Source: CAD feature listing. Evaluate the final solid. Frame: model axes, mm. A direction names the side the tool comes from. Coordinates: 2 decimals unless noted, no trailing zeros. Order: outer loops, then holes, each group sorted by start corner. A loop starts at its lowest first (then second) coordinate and runs counter-clockwise, first axis right, second up.
```python
from build123d import *

# Parameters (mm, degrees)
SKETCH2_W            = 45.5
SKETCH2_H            = 21
BOSS_EXTRUDE2_DEPTH  = 2
SKETCH4_R            = 8
BOSS_EXTRUDE3_DEPTH  = 12.5
SKETCH5_R            = 6
CUT_EXTRUDE1_DEPTH   = 2.5
BOSS_EXTRUDE5_DEPTH  = 4
SKETCH7_W            = 6
SKETCH7_H            = 3
BOSS_EXTRUDE6_DEPTH  = 3
SKETCH8_W            = 1
SKETCH8_H            = 1
BOSS_EXTRUDE7_DEPTH  = 1
SKETCH10_W           = 1
SKETCH10_H           = 0.8
BOSS_EXTRUDE8_DEPTH  = 6
SKETCH11_R           = 1
CUT_EXTRUDE2_DEPTH   = 15.5
BOSS_EXTRUDE10_DEPTH = 0.1


with BuildPart() as part:
    # Sketch2 → Boss-Extrude2 (new body)
    with BuildSketch(Plane(origin=(0, 0, 0), x_dir=(1, 0, 0), z_dir=(0, 1, 0))):
        with Locations((-22.75, 10.5)):
            Rectangle(SKETCH2_W, SKETCH2_H)
    extrude(amount=BOSS_EXTRUDE2_DEPTH)

    # Sketch4 → Boss-Extrude3 (add)
    with BuildSketch(Plane(origin=(0, 2, 0), x_dir=(1, 0, 0), z_dir=(0, 1, 0))):
        with Locations((-35, 10.5)):
            Circle(SKETCH4_R)
        with Locations((-10.5, 10.5)):
            Circle(SKETCH4_R)
    extrude(amount=BOSS_EXTRUDE3_DEPTH)

    # Sketch5 → Cut-Extrude1 (cut)
    with BuildSketch(Plane(origin=(0, 14.5, 0), x_dir=(1, 0, 0), z_dir=(0, 1, 0))):
        with Locations((-35, 10.5)):
            Circle(SKETCH5_R)
        with Locations((-10.5, 10.5)):
            Circle(SKETCH5_R)
    extrude(amount=-CUT_EXTRUDE1_DEPTH, mode=Mode.SUBTRACT)

    # Sketch6 → Boss-Extrude5 (add)
    with BuildSketch(Plane(origin=(0, 2, 0), x_dir=(1, 0, 0), z_dir=(0, 1, 0))):
        with BuildLine():
            Line((-25.75, 20.493953902), (-19.75, 20.493953902))
            ThreePointArc((-19.75, 20.493953902), (-17.756046098, 18.5), (-19.75, 16.506046098))
            Line((-19.75, 16.506046098), (-25.75, 16.506046098))
            ThreePointArc((-25.75, 16.506046098), (-27.743953902, 18.5), (-25.75, 20.493953902))
        make_face()
    extrude(amount=BOSS_EXTRUDE5_DEPTH)

    # Sketch7 → Boss-Extrude6 (add)
    with BuildSketch(Plane.XZ):
        with Locations((-19.75, -1.5)):
            Rectangle(SKETCH7_W, SKETCH7_H)
        with Locations((-25.75, -1.5)):
            Rectangle(SKETCH7_W, SKETCH7_H)
    extrude(amount=BOSS_EXTRUDE6_DEPTH)

    # Sketch8 → Boss-Extrude7 (add)
    with BuildSketch(Plane.XZ.offset(3)):
        with Locations((-24.25, -1.5)):
            Rectangle(SKETCH8_W, SKETCH8_H)
        with Locations((-21.25, -1.5)):
            Rectangle(SKETCH8_W, SKETCH8_H)
        with Locations((-18.25, -1.5)):
            Rectangle(SKETCH8_W, SKETCH8_H)
        with Locations((-27.25, -1.5)):
            Rectangle(SKETCH8_W, SKETCH8_H)
    extrude(amount=BOSS_EXTRUDE7_DEPTH)

    # Sketch10 → Boss-Extrude8 (add)
    with BuildSketch(Plane.XY.offset(-1)):
        with Locations((-18.25, -3.6)):
            Rectangle(SKETCH10_W, SKETCH10_H)
        with Locations((-21.25, -3.6)):
            Rectangle(SKETCH10_W, SKETCH10_H)
        with Locations((-24.25, -3.6)):
            Rectangle(SKETCH10_W, SKETCH10_H)
        with Locations((-27.25, -3.6)):
            Rectangle(SKETCH10_W, SKETCH10_H)
    extrude(amount=BOSS_EXTRUDE8_DEPTH)

    # Sketch11 → Cut-Extrude2 (cut, through all)
    with BuildSketch(Plane.XZ):
        with Locations((-2, -19)):
            Circle(SKETCH11_R)
        with Locations((-43.5, -2)):
            Circle(SKETCH11_R)
    extrude(amount=-CUT_EXTRUDE2_DEPTH, mode=Mode.SUBTRACT)

    # Sketch15 → Boss-Extrude10 (add)
    with BuildSketch(Plane(origin=(0, 2, 0), x_dir=(1, 0, 0), z_dir=(0, 1, 0))):
        Polygon((-41.795833333, 3.38023745), (-41.795833333, 3.705878476), (-40.126923077, 3.705878476), (-40.126923077, 3.38023745), (-40.818910256, 3.38023745), (-40.818910256, 0.530878476), (-41.103846154, 0.530878476), (-41.103846154, 3.38023745), align=None)
        with BuildLine():
            Line((-5.446153846, 3.705878476), (-4.810772236, 3.705878476))
            add(Edge.make_bspline(
                [(-4.810772236, 3.705878476), (-4.768371355, 3.705737337), (-4.686956967, 3.705466335), (-4.570322643, 3.70395525), (-4.464343776, 3.699624228), (-4.369075779, 3.695897155), (-4.284520399, 3.689100894), (-4.210418357, 3.682605164), (-4.147110946, 3.674101915), (-4.108787923, 3.666204853), (-4.091436298, 3.662629277)],
                knots=[0, 0, 0, 0, 0.000127205, 0.000244248, 0.000349896, 0.000445402, 0.000530231, 0.00060434, 0.000668562, 0.000721699, 0.000721699, 0.000721699, 0.000721699], degree=3))
            add(Edge.make_bspline(
                [(-4.091436298, 3.662629277), (-4.068207432, 3.656889997), (-4.022245234, 3.645533872), (-3.956069103, 3.621531234), (-3.893009681, 3.59375486), (-3.833328911, 3.561130628), (-3.777325729, 3.523416363), (-3.72442269, 3.481263138), (-3.674379734, 3.434901601), (-3.629220684, 3.383162852), (-3.586640258, 3.32888259), (-3.550727719, 3.270187039), (-3.519770126, 3.208808368), (-3.495122586, 3.144122353), (-3.475276139, 3.076756317), (-3.461282336, 3.006100052), (-3.452890187, 2.932475453), (-3.452035789, 2.882257921), (-3.451602564, 2.856794942)],
                knots=[0, 0, 0, 0, 7.1738e-05, 0.000141945, 0.000210849, 0.000278309, 0.000345694, 0.000413139, 0.000481086, 0.000550014, 0.000618962, 0.000687796, 0.000756061, 0.000824921, 0.000895163, 0.000966511, 0.001040751, 0.001117115, 0.001117115, 0.001117115, 0.001117115], degree=3))
            add(Edge.make_bspline(
                [(-3.451602564, 2.856794942), (-3.452935155, 2.81449024), (-3.455535386, 2.731942809), (-3.479778873, 2.612144724), (-3.51949043, 2.500394417), (-3.574212271, 2.396832596), (-3.643898509, 2.303477939), (-3.727650284, 2.221480883), (-3.825514317, 2.152864676), (-3.916618054, 2.105282489), (-3.997094506, 2.074808922), (-4.063346155, 2.053367368), (-4.135615484, 2.036801157), (-4.213210066, 2.02196018), (-4.296452811, 2.010755429), (-4.385144204, 2.002548875), (-4.479347498, 1.997419845), (-4.544062226, 1.996656027), (-4.577353766, 1.996263091)],
                knots=[0, 0, 0, 0, 0.000126797, 0.000247415, 0.000364897, 0.000481551, 0.000597433, 0.000713022, 0.000831615, 0.000954788, 0.001020224, 0.001089619, 0.001163513, 0.001242474, 0.001326575, 0.001415367, 0.001509635, 0.001609508, 0.001609508, 0.001609508, 0.001609508], degree=3))
            Line((-4.577353766, 1.996263091), (-3.410897436, 0.530878476))
            Line((-3.410897436, 0.530878476), (-3.763251202, 0.530878476))
            Line((-3.763251202, 0.530878476), (-4.929707532, 1.996263091))
            Line((-4.929707532, 1.996263091), (-5.161217949, 1.996263091))
            Line((-5.161217949, 1.996263091), (-5.161217949, 0.530878476))
            Line((-5.161217949, 0.530878476), (-5.446153846, 0.530878476))
            Line((-5.446153846, 0.530878476), (-5.446153846, 3.705878476))
        make_face()
        with BuildLine():
            Line((-5.161217949, 3.38023745), (-5.161217949, 2.321904117))
            Line((-5.161217949, 2.321904117), (-4.579897837, 2.317451994))
            add(Edge.make_bspline(
                [(-4.579897837, 2.317451994), (-4.552756087, 2.317439986), (-4.500147646, 2.317416712), (-4.424037757, 2.321039638), (-4.353171656, 2.325161076), (-4.287820402, 2.331465125), (-4.227954802, 2.339589562), (-4.173604777, 2.349752269), (-4.124681608, 2.361592354), (-4.067623648, 2.379918115), (-4.003909081, 2.408952146), (-3.934665542, 2.451193705), (-3.875699136, 2.504324263), (-3.825880789, 2.565078756), (-3.785849091, 2.631877353), (-3.757626013, 2.703919345), (-3.739716797, 2.779386009), (-3.737604474, 2.831254721), (-3.736538462, 2.85743096)],
                knots=[0, 0, 0, 0, 8.1413e-05, 0.000157801, 0.000228539, 0.000294357, 0.000354712, 0.000409723, 0.000460165, 0.000505621, 0.000589315, 0.00066961, 0.000747992, 0.000826171, 0.000904597, 0.000980539, 0.001057529, 0.001135968, 0.001135968, 0.001135968, 0.001135968], degree=3))
            add(Edge.make_bspline(
                [(-3.736538462, 2.85743096), (-3.737628957, 2.882963923), (-3.739789921, 2.93356094), (-3.757432733, 3.007634515), (-3.7872681, 3.077545249), (-3.827474702, 3.143008746), (-3.876459649, 3.202431806), (-3.933897951, 3.253274581), (-3.998219092, 3.295229452), (-4.058336537, 3.322039498), (-4.112070429, 3.338476793), (-4.158724478, 3.35004392), (-4.21143989, 3.359337117), (-4.270472627, 3.366783001), (-4.335570678, 3.373182843), (-4.407063197, 3.377493385), (-4.484475848, 3.380045962), (-4.538130564, 3.380172135), (-4.565905449, 3.38023745)],
                knots=[0, 0, 0, 0, 7.6536e-05, 0.000151667, 0.000226914, 0.000303706, 0.000381394, 0.000457083, 0.00053294, 0.00061095, 0.000653596, 0.000701416, 0.000755061, 0.00081407, 0.000879888, 0.000951261, 0.001028897, 0.001112218, 0.001112218, 0.001112218, 0.001112218], degree=3))
            Line((-4.565905449, 3.38023745), (-5.161217949, 3.38023745))
        make_face(mode=Mode.SUBTRACT)
    extrude(amount=BOSS_EXTRUDE10_DEPTH)


solid = part.part
```
1. Pin query (flat end, axial travel): P1, Ø6, axis at x = -22, y = 2, coming from the +Z side; P2, Ø10.5, axis at x = -14, z = -9, coming from the -Y side; P3, Ø1.5, axis at x = -27, z = 0.5, coming from the +Y side. Return the tip coordinate at first contact, or that it passes through.
Findings:
P1: stops at z = 0
P2: stops at y = 0
P3: stops at y = 2
2. Access query for faces 1 (the face through (-23.75, -3.6, 1.5)), 2 (the face through (-21, -3.2, 2)), 3 (the face through (-23, 4, -16.506)). Directions: +Z, -Z, +X, -X, +Y, -Y. A direction counts if a zero-diameter tool reaches every point of the face in a straight line with its end or side. Return the directions, or none.
Findings:
face 1: +Z, -Z, -Y
face 2: +Z, +X, -X
face 3: +Z, +Y
3. Draft query along X for faces 4 (the face through (-16.75, -1, -2)), 5 (the face through (-24.75, -3.6, 1.5)), 6 (the face through (-24.3, -3.5, -2)). Return one class per face: released by +X, released by -X, zero draft, split by the parting line, or undercut.
Findings:
face 4: released by +X
face 5: undercut
face 6: zero draft
4. Section query A-A on x = -43.5. Return loops of the section in (y, z), plus the area to 3 significant figures.
Findings:
outline: (0, -21) - (2, -21) - (2, -3) - (0, -3) - close; (0, -1) - (2, -1) - (2, 0) - (0, 0) - close
area: 38.0 mm2
5. Ray query, line 1 (X direction, y = 12.9, z = -10.5); line 2 (X direction, y = 13.5, z = -7.75); line 3 (Y direction, x = -44, z = -13). Return the intervals inside material, ascending.
Findings:
line 1: x = -43 to -41, -29 to -27, -18.5 to -16.5, -4.5 to -2.5
line 2: x = -42.51 to -40.33, -29.67 to -27.49, -18.01 to -15.83, -5.17 to -2.99
line 3: y = 0 to 2
6. Section query C-C on z = -10.5. Return loops of the section in (x, y).
Findings:
outline: (-45.5, 0) - (0, 0) - (0, 2) - (-2.5, 2) - (-2.5, 14.5) - (-4.5, 14.5) - (-4.5, 12) - (-16.5, 12) - (-16.5, 14.5) - (-18.5, 14.5) - (-18.5, 2) - (-27, 2) - (-27, 14.5) - (-29, 14.5) - (-29, 12) - (-41, 12) - (-41, 14.5) - (-43, 14.5) - (-43, 2) - (-45.5, 2) - close
7. Section query B-B on y = 3.5. Return loops of the section in (x, z), plus the area to 3 significant figures.
Findings:
outline: circle Ø16 at (-35, -10.5); (-25.75, -20.49) - (-19.75, -20.49) arc R1.99 ccw to (-19.75, -16.51) - (-25.75, -16.51) arc R1.99 ccw to start; circle Ø16 at (-10.5, -10.5)
area: 439 mm2
8. Section query D-D on x = -10.5. Return loops of the section in (y, z).
Findings:
outline: (0, -21) - (2, -21) - (2, -18.5) - (14.5, -18.5) - (14.5, -16.5) - (12, -16.5) - (12, -4.5) - (14.5, -4.5) - (14.5, -2.5) - (2, -2.5) - (2, 0) - (0, 0) - close
